Part model, mm, in its own coordinate system. Face numbers are marked on the shaded views. A direction names the side the tool comes from. Give positions to 0.01 mm unless a question says otherwise; leave off trailing zeros. Loops run counter-clockwise (first coordinate to the right, second up) from the corner with the lowest first, then second, coordinate; pieces in that order, holes last. Notation, with made-up numbers: (27.5, 23.25) -> (84.5, 23.25) arc R18 ccw to (84.5, 28.25) -> close; hole circle Ø1 at (-1.75, -18.75). An arc over 180 degrees is marked (long way). One line per question, with ' | ' between items.
Autodesk Inventor part; units mm, degrees
ref_plane "Work Plane1" through (4.625, 0, 0) normal (0, 0, -1) x (1, 0, 0)
ref_plane "YZ Plane" through (0, 0, 0) normal (1, 0, 0) x (0, 1, 0)
ref_plane "XZ Plane" through (0, 0, 0) normal (0, 1, 0) x (-1, 0, 0)
sketch "Sketch1" plane through (0, 0, 0) normal (0, 0, 1) x (1, 0, 0)
  line L0 (0, 0) -> (8, 0)
  line L1 (8, 0) -> (8, 1)
  line L2 (8, 1) -> (1.25, 1)
  line L3 (0, -0.2) -> (0, 1.2)
  line L4 (0, 0.5) -> (0, 0)
  line L5 (0, 0.5) -> (1.25, 0.5)
  line L6 (1.25, 0.5) -> (1.25, 1)
  dimension "d1" = 8
  dimension "d2" = 1
  dimension "d13" = 2
  dimension "d14" = 1.25
revolve "Body" add sketch "Sketch1" angle 360 about axis through (0, 0, 0) along (1, 0, 0)
chamfer "Chamfer1" distance 0.2454 angle 45 1 edges at (8, -1, 0) measured on face at (8, -0.1923, -0.0109)
sketch "Sketch2" plane through (0, 0, 0) normal (0, 0, 1) x (1, 0, 0)
  line L0 (8, 0.7546) -> (8, -0.7546)
  line L1 (7.232, 0) -> (8.128, 0)
  line L2 (8, 0.125) -> (7.36, 0.125)
  line L3 (7.36, 0.125) -> (7.36, 0)
  line L4 (7.36, -0.125) -> (7.36, 0)
  line L5 (7.36, -0.125) -> (8, -0.125)
  dimension "d8" = 0.125
  dimension "d9" = 0.64
extrude "Slot" cut sketch "Sketch2" against normal mid plane 2
thread "Thread"
chamfer "Chamfer2" distance 0.5 angle 45 1 edges at (1.25, -1, 0) measured on face at (1.25, 0.8236, -0.0798)
ref_plane "Work Plane1" through (4.625, 0, 0) normal (0, 0, -1) x (1, 0, 0)
equation "\"d8\" = 0.5 * SBR"
equation "\"d9\" = STI"
equation "\"d10\" = NND"
equation "\"d3\" = -0.5 * GD1 + 0.5 * NND"
equation "\"d4\" = FAWI"
equation "\"d37\" = -0.5 * GD1 + 0.5 * NND"
equation "\"d5\" = NLG - ZLG"
equation "\"d15\" = -0.5 * SPD + 0.5 * NND"
equation "\"d16\" = FAWI"
equation "\"d38\" = -0.5 * SPD + 0.5 * NND"
equation "\"d1\" = NLG"
equation "\"d2\" = SPD"
equation "\"d13\" = NND"
equation "\"d14\" = ZLG"
equation "\"NND\" = 2"
equation "\"NLG\" = 8"
equation "\"FAWI\" = 45deg"
equation "\"GD1\" = THREADDIA - 1.2269 * PTC"
equation "\"FAWI1\" = 45deg"
equation "\"SPD\" = 1"
equation "\"SBR\" = 0.25"
equation "\"STI\" = 0.64"
equation "\"ZLG\" = 1.25"
equation "\"GUL\" = 0.61345 * PTC"
equation "\"THREADDIA\" = 2"
equation "\"TOA\" = 30deg"
equation "\"PTC\" = 0.4"
equation "\"GAL\" = 0.61345 * PTC"
properties part number "ISO 7435 - M2 x 8" material "Stainless Steel, 440C"
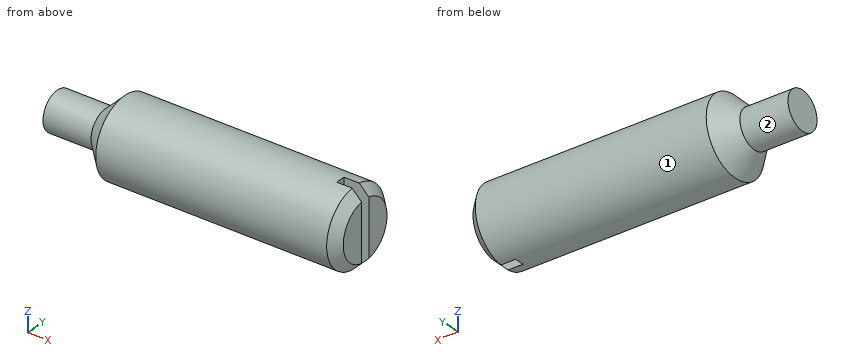
1) Drill centre lines: line 1 (Y direction, x = 6, z = -0.05); line 2 (X direction, y = 0, z = 0.3); line 3 (X direction, y = 0.9, z = -0.05). Where is each one in solid material? Low to high.
Found:
line 1: -1 to 1 | line 2: 0 to 7.36 | line 3: 1.65 to 7.85
2) Tool access for the marked faces 1 and 2: list every direction of +Z, -Z, +X, -X, +Y, -Y with a clear straight run to the whole face (end or side of a thin tool).
Found:
face 1: +X, -X | face 2: -X
3) Saw through at C-C (x = 5). Give the cut face in (y, z).
Found:
outline: circle Ø2 at (0, 0)
